Geometry check sheet. Reference: the model listing, model coordinates, mm. Give positions to 0.01 mm unless a question says otherwise; leave off trailing zeros. Loops run counter-clockwise (first coordinate to the right, second up) from the corner with the lowest first, then second, coordinate; pieces in that order, holes last. Notation, with made-up numbers: (-0.75, 73.5) -> (31.25, 73.5) arc R27 cw to (31.25, 112.5) -> close; hole circle Ø3 at (89.5, 58). An arc over 180 degrees is marked (long way). One line per item, written item: value. Start each with the question number.
(1) Draft check along Z on faces 1 (the face through (-1, 0, -1)), 2 (the face through (54.464, 1.014, 55.125)). Enter one of: pulls with the +Z half, pulls with the -Z half, needs draft (parallel to the pull), parting line crosses it, or undercut.
(2) Scan lines: line 1 along X through (y, z) = (1.35, 55); line 2 along X through (y, z) = (0.85, 50); line 3 along Z through (x, y) = (39.5, 1.3). Record each from-to range of solid material in increasing order. Write a range as from..to.
(3) Sectioned sample at B-B, the plane x = 6. Record the cut outline in (y, z), then the cut area to 3 significant figures.
(4) Sectioned sample at C-C, the plane x = 53. Record the cut outline in (y, z) (3 decimals), then the cut area to 3 significant figures.
(5) Gauge pin test, flat ends, axial feed: pin 1 Ø4 at (x, z) = (-25, 29.63) entering from +Y; pin 2 Ø2.5 at (x, z) = (-53, -54) entering from -Y. Record the tip position at first contact, or that the pin passes through.
(6) Sectioned sample at D-D, the plane y = 1.35. State how many separate pieces and enclosed holes the cut face has, then the cut area to 3 significant figures.
(7) Sectioned sample at A-A, the plane z = -37.5. Record the cut outline in (x, y).
from build123d import *

# Parameters (mm, degrees)
SKETCH1_W           = 120
SKETCH1_H           = 120
BOSS_EXTRUDE1_DEPTH = 2
SKETCH2_R           = 1.525
SKETCH2_R_2         = 1.5
CUT_EXTRUDE1_DEPTH  = 2
SKETCH4_R           = 1.5
SKETCH4_R_2         = 1.55
SKETCH4_W           = 12
SKETCH4_H           = 60
CUT_EXTRUDE2_DEPTH  = 85.876380696
SKETCH5_R           = 1.5
SKETCH5_W           = 30
SKETCH5_H           = 2.5
CUT_EXTRUDE3_DEPTH  = 85.876380696


with BuildPart() as part:
    # Sketch1 → Boss-Extrude1 (new body)
    with BuildSketch(Plane(origin=(0, 0, 0), x_dir=(1, 0, 0), z_dir=(0, 1, 0))):
        Rectangle(SKETCH1_W, SKETCH1_H)
    extrude(amount=BOSS_EXTRUDE1_DEPTH)

    # Sketch2 → Cut-Extrude1 (cut)
    with BuildSketch(Plane(origin=(0, 2, 0), x_dir=(1, 0, 0), z_dir=(0, 1, 0))):
        with Locations(Location((-53, 54, 0), (0, 0, 270))):
            Circle(SKETCH2_R)
        with Locations(Location((-53, -54.8, 0), (0, 0, 270))):
            Circle(SKETCH2_R_2)
        with Locations(Location((53, 54, 0), (0, 0, 90))):
            Circle(SKETCH2_R)
        with Locations(Location((53, -54.8, 0), (0, 0, 90))):
            Circle(SKETCH2_R_2)
    extrude(amount=-CUT_EXTRUDE1_DEPTH, mode=Mode.SUBTRACT)

    # Sketch4 → Cut-Extrude2 (cut, through all)
    with BuildSketch(Plane(origin=(0, 2, 0), x_dir=(1, 0, 0), z_dir=(0, 1, 0))):
        with Locations(Location((-25, 53, 0), (0, 0, 270))):
            Circle(SKETCH4_R)
        with Locations(Location((-25, -29.63, 0), (0, 0, 270))):
            Circle(SKETCH4_R)
        with Locations(Location((23.34, -22.13, 0), (0, 0, 270))):
            Circle(SKETCH4_R_2)
        with Locations((-42, 20)):
            Rectangle(SKETCH4_W, SKETCH4_H)
        with Locations((42, 20)):
            Rectangle(SKETCH4_W, SKETCH4_H)
    extrude(amount=-CUT_EXTRUDE2_DEPTH, mode=Mode.SUBTRACT)

    # Sketch5 → Cut-Extrude3 (cut, through all)
    with BuildSketch(Plane(origin=(0, 2, 0), x_dir=(1, 0, 0), z_dir=(0, 1, 0))):
        with Locations(Location((-54, -45, 0), (0, 0, 270))):
            Circle(SKETCH5_R)
        with Locations(Location((-28.82, -45, 0), (0, 0, 270))):
            Circle(SKETCH5_R)
        with Locations(Location((-54, -21.9, 0), (0, 0, 270))):
            Circle(SKETCH5_R)
        with Locations(Location((24.479587092, -50, 0), (0, 0, 270))):
            Circle(SKETCH5_R)
        with Locations(Location((39.479587092, -50, 0), (0, 0, 270))):
            Circle(SKETCH5_R)
        with Locations((0, -56.75)):
            Rectangle(SKETCH5_W, SKETCH5_H)
    extrude(amount=-CUT_EXTRUDE3_DEPTH, mode=Mode.SUBTRACT)


solid = part.part
Calculated:
1. face 1: needs draft
1. face 2: undercut
2. line 1: x = -60..-54.49, -51.51..51.51, 54.49..60
2. line 2: x = -60..22.98, 25.98..37.98, 40.98..60
2. line 3: z = -60..-50, 10..48.5, 51.5..60
3. outline: (0, -60) -> (2, -60) -> (2, 55.5) -> (0, 55.5) -> close; (0, 58) -> (2, 58) -> (2, 60) -> (0, 60) -> close
3. area: 235 mm2
4. outline: (0, -60) -> (2, -60) -> (2, -55.525) -> (0, -55.525) -> close; (0, -52.475) -> (2, -52.475) -> (2, 53.3) -> (0, 53.3) -> close; (0, 56.3) -> (2, 56.3) -> (2, 60) -> (0, 60) -> close
4. area: 228 mm2
5. pin 1: stops at y = 2
5. pin 2: passes through
6. separate pieces: 1
6. enclosed holes: 15
6. area: 12,800 mm2
7. outline: (-60, 0) -> (-48, 0) -> (-48, 2) -> (-60, 2) -> close; (-36, 0) -> (36, 0) -> (36, 2) -> (-36, 2) -> close; (48, 0) -> (60, 0) -> (60, 2) -> (48, 2) -> close
